```python
from build123d import *

# Parameters (mm, degrees)
F0_R            = 33.02
F0_R_2          = 23.495
F1_DEPTH        = 7.62
F3_DEPTH        = 5.08
F3_COPIES_COUNT = 18


# Not quite as in the source:
# - a pattern or mirror of a feature is missing from the dataset's text; its kind, count and spacing are read off the source's solid


with BuildPart() as f1:
    # F0 (on Top) → F1 (new body)
    with BuildSketch(Plane.XY):
        Circle(F0_R)
        Circle(F0_R_2, mode=Mode.SUBTRACT)
    extrude(amount=F1_DEPTH)

    # F2 (on face) → F3 (cut)
    with BuildSketch(Plane.XY.offset(7.62)):
        with BuildLine():
            Line((-3.4519625326, -29.1909987132), (-3.4519625326, -32.8390675061))
            ThreePointArc((-3.4519625326, -32.8390675061), (-1.1687703181, -32.9993087192), (1.1200374674, -33.0009987132))
            Line((1.1200374674, -33.0009987132), (1.1200374674, -29.1909987132))
            Line((1.1200374674, -29.1909987132), (-3.4519625326, -29.1909987132))
        make_face()
    f3 = extrude(amount=-F3_DEPTH, mode=Mode.SUBTRACT)

    # F3_copies: F3 ×18 about axis
    f3_copies_axis = Axis((0, 0, 0), (0, 0, 1))
    for i in range(1, F3_COPIES_COUNT):
        add(f3.rotate(f3_copies_axis, i * 360 / F3_COPIES_COUNT), mode=Mode.SUBTRACT)


solid = f1.part
```
Source: CAD feature listing. Evaluate the final solid. Frame: model axes, mm. A direction names the side the tool comes from. Round coordinates to 2 decimals unless told otherwise and drop trailing zeros. Loops run counter-clockwise (first coordinate to the right, second up) from the corner with the lowest first, then second, coordinate; pieces in that order, holes last.
1. Section query B-B on y = 0. Output: boundary loops of the cut face in (x, z) (3 decimals).
2. Ray query, L1, parallel to Y at x = 0, z = 4.5 (3 decimals); L2, parallel to X at y = 15, z = 4.25; L3, parallel to X at y = -21, z = 5.75. Return the intervals inside material, ascending.
3. Access query for faces 4 (the flat face through (-21, -23, 2.54)), 5 (the flat face through (26.39, 16.53, 5.12)), 6 (the flat face through (-1.12, 31, 5)). Directions: +Z, -Z, +X, -X, +Y, -Y. A direction counts if a zero-diameter tool reaches every point of the face in a straight line with its end or side. Return the directions, or none.
4. Section query A-A on x = 0. Output: boundary loops of the cut face in (y, z) (3 decimals), and give its area (3 significant figures).
5. Section query C-C on y = -18.5. Output: boundary loops of the cut face in (x, z).
6. Mould query, pull axis X, two halves, no side actions, for faces 1 (the flat face through (29.92, -8.78, 5.12)), 2 (the flat face through (-29.92, 8.78, 5.12)), 3 (the flat face through (19, -25, 2.54)). Classes: released by +X, released by -X, zero draft, split by the parting line, or undercut.
7. Contact query for flat-ended pins moving along their axis: pin 1 (2.5 mm diameter, centred on x = 0.5, z = 4, fed in from +Y); pin 2 (3 mm diameter, centred on x = 20.5, y = -10.5, fed in from +Z); pin 3 (3 mm diameter, centred on x = 2, z = 6.5, fed in from -Y); pin 4 (2 mm diameter, centred on x = -16.5, z = 3.5, fed in from -Y). Output: stop coordinate, or through.
Answers below:
1. outline: (-33.02, 0) - (-23.495, 0) - (-23.495, 7.62) - (-33.02, 7.62) - close; (23.495, 0) - (33.02, 0) - (33.02, 7.62) - (23.495, 7.62) - close
2. L1: y = -29.191 to -23.495, 23.495 to 29.191
2. L2: x = -29.42 to -28.22, -25.05 to -18.08, 18.08 to 25.05
2. L3: x = -25.48 to -22.13, -20.39 to -10.54, 10.54 to 25.48
3. face 4: +Z
3. face 5: +Z, +X
3. face 6: +Z, +Y
4. outline: (-33.02, 0) - (-23.495, 0) - (-23.495, 7.62) - (-29.191, 7.62) - (-29.191, 2.54) - (-33.02, 2.54) - close; (23.495, 0) - (33.02, 0) - (33.02, 2.54) - (29.191, 2.54) - (29.191, 7.62) - (23.495, 7.62) - close
4. area: 106 mm2
5. outline: (-27.35, 0) - (-14.48, 0) - (-14.48, 7.62) - (-27.35, 7.62) - close; (14.48, 0) - (27.35, 0) - (27.35, 2.54) - (25.14, 2.54) - (25.14, 7.62) - (14.48, 7.62) - close
6. face 1: released by +X
6. face 2: released by -X
6. face 3: undercut
7. pin 1: stops at y = 29.19
7. pin 2: stops at z = 7.62
7. pin 3: stops at y = -33
7. pin 4: stops at y = -29.16
